from build123d import *

# Parameters (mm, degrees)
SKETCH1_W           = 153.67
SKETCH1_H           = 77.47
SKETCH1_R           = 2.667
SKETCH1_R_2         = 3.683
BOSS_EXTRUDE1_DEPTH = 6.096


with BuildPart() as part:
    # Sketch1 → Boss-Extrude1 (new body)
    with BuildSketch(Plane(origin=(0, 0, 0), x_dir=(1, 0, 0), z_dir=(0, 1, 0))):
        Rectangle(SKETCH1_W, SKETCH1_H)
        with Locations((-68.072, 29.972)):
            Circle(SKETCH1_R, mode=Mode.SUBTRACT)
        with Locations((-68.072, 14.732)):
            Circle(SKETCH1_R, mode=Mode.SUBTRACT)
        with Locations((-68.072, 0)):
            Circle(SKETCH1_R, mode=Mode.SUBTRACT)
        with Locations((-68.072, -29.972)):
            Circle(SKETCH1_R, mode=Mode.SUBTRACT)
        with Locations((-68.072, -16.256)):
            Circle(SKETCH1_R_2, mode=Mode.SUBTRACT)
        with Locations((-47.752, -29.972)):
            Circle(SKETCH1_R, mode=Mode.SUBTRACT)
        with Locations((-47.752, -16.256)):
            Circle(SKETCH1_R_2, mode=Mode.SUBTRACT)
        with Locations((-47.752, 0)):
            Circle(SKETCH1_R, mode=Mode.SUBTRACT)
        with Locations((-47.752, 14.732)):
            Circle(SKETCH1_R, mode=Mode.SUBTRACT)
        with Locations((-47.752, 29.972)):
            Circle(SKETCH1_R, mode=Mode.SUBTRACT)
        with Locations((-29.21, 29.972)):
            Circle(SKETCH1_R, mode=Mode.SUBTRACT)
        with Locations((-8.89, 29.972)):
            Circle(SKETCH1_R, mode=Mode.SUBTRACT)
        with Locations((-29.21, 8.89)):
            Circle(SKETCH1_R, mode=Mode.SUBTRACT)
        with Locations((-29.21, -8.89)):
            Circle(SKETCH1_R, mode=Mode.SUBTRACT)
        with Locations((-8.89, -29.972)):
            Circle(SKETCH1_R, mode=Mode.SUBTRACT)
        with Locations((-29.21, -29.972)):
            Circle(SKETCH1_R, mode=Mode.SUBTRACT)
        with Locations((-57.912, 20.066)):
            Circle(SKETCH1_R, mode=Mode.SUBTRACT)
        with Locations((-57.912, -20.066)):
            Circle(SKETCH1_R, mode=Mode.SUBTRACT)
        with Locations((-20.32, 20.066)):
            Circle(SKETCH1_R, mode=Mode.SUBTRACT)
        with Locations((-20.32, -20.066)):
            Circle(SKETCH1_R, mode=Mode.SUBTRACT)
        with Locations((-38.862, 20.066)):
            Circle(SKETCH1_R, mode=Mode.SUBTRACT)
        with Locations((-38.862, -20.066)):
            Circle(SKETCH1_R, mode=Mode.SUBTRACT)
        with Locations((20.32, -20.066)):
            Circle(SKETCH1_R, mode=Mode.SUBTRACT)
        with Locations((8.89, -29.972)):
            Circle(SKETCH1_R, mode=Mode.SUBTRACT)
        with Locations((29.21, -29.972)):
            Circle(SKETCH1_R, mode=Mode.SUBTRACT)
        with Locations((38.862, -20.066)):
            Circle(SKETCH1_R, mode=Mode.SUBTRACT)
        with Locations((47.752, -29.972)):
            Circle(SKETCH1_R, mode=Mode.SUBTRACT)
        with Locations((68.072, -29.972)):
            Circle(SKETCH1_R, mode=Mode.SUBTRACT)
        with Locations((68.072, 0)):
            Circle(SKETCH1_R, mode=Mode.SUBTRACT)
        with Locations((68.072, -16.256)):
            Circle(SKETCH1_R_2, mode=Mode.SUBTRACT)
        with Locations((57.912, -20.066)):
            Circle(SKETCH1_R, mode=Mode.SUBTRACT)
        with Locations((47.752, -16.256)):
            Circle(SKETCH1_R_2, mode=Mode.SUBTRACT)
        with Locations((29.21, -8.89)):
            Circle(SKETCH1_R, mode=Mode.SUBTRACT)
        with Locations((29.21, 8.89)):
            Circle(SKETCH1_R, mode=Mode.SUBTRACT)
        with Locations((57.912, 20.066)):
            Circle(SKETCH1_R, mode=Mode.SUBTRACT)
        with Locations((68.072, 14.732)):
            Circle(SKETCH1_R, mode=Mode.SUBTRACT)
        with Locations((68.072, 29.972)):
            Circle(SKETCH1_R, mode=Mode.SUBTRACT)
        with Locations((47.752, 14.732)):
            Circle(SKETCH1_R, mode=Mode.SUBTRACT)
        with Locations((47.752, 0)):
            Circle(SKETCH1_R, mode=Mode.SUBTRACT)
        with Locations((38.862, 20.066)):
            Circle(SKETCH1_R, mode=Mode.SUBTRACT)
        with Locations((20.32, 20.066)):
            Circle(SKETCH1_R, mode=Mode.SUBTRACT)
        with Locations((8.89, 29.972)):
            Circle(SKETCH1_R, mode=Mode.SUBTRACT)
        with Locations((29.21, 29.972)):
            Circle(SKETCH1_R, mode=Mode.SUBTRACT)
        with Locations((47.752, 29.972)):
            Circle(SKETCH1_R, mode=Mode.SUBTRACT)
        with BuildLine():
            Line((13.716, 14.986), (-13.716, 14.986))
            ThreePointArc((-13.716, 14.986), (-18.206128061, 13.126128061), (-20.066, 8.636))
            Line((-20.066, 8.636), (-20.066, -8.636))
            ThreePointArc((-20.066, -8.636), (-18.206128061, -13.126128061), (-13.716, -14.986))
            Line((-13.716, -14.986), (13.716, -14.986))
            ThreePointArc((13.716, -14.986), (18.206128061, -13.126128061), (20.066, -8.636))
            Line((20.066, -8.636), (20.066, 8.636))
            ThreePointArc((20.066, 8.636), (18.206128061, 13.126128061), (13.716, 14.986))
        make_face(mode=Mode.SUBTRACT)
    extrude(amount=BOSS_EXTRUDE1_DEPTH)


solid = part.part
Design review of the part built by this model. Coordinates are the model's own, in mm. A direction names the side the tool comes from. Coordinates: 2 decimals unless noted, no trailing zeros. Loops run counter-clockwise (first coordinate to the right, second up) from the corner with the lowest first, then second, coordinate; pieces in that order, holes last. Notation, with made-up numbers: (82, 38.25) -> (141, 38.25) arc R36 cw to (141, 74.25) -> close; hole circle Ø11 at (85.25, 37). An arc over 180 degrees is marked (long way). Use a Markdown table: item, result. Add a question column.
Item 1: Machinability: for faces 4 (the flat face through (20.066, 3, 0)), 5 (the flat face through (-1, 6.096, -18)), which of the approach directions +Z, -Z, +X, -X, +Y, -Y give a long, thin tool a straight path to every point of the face, cutting with its end or side? Answer none if there is none.
Item 2: We need section B-B, the plane z = 0. Write out the cut boundary in (x, y) (3 decimals), and give its area (3 significant figures).
Item 3: The part is to be moulded in two halves that separate along Z. For faces 1 (the flat face through (-76.835, 3, 1)), 2 (the cylindrical face through (49.19, 3.01, -32.22)), 3 (the cylindrical face through (36.746, 3.005, 21.689)), say which applies: +Z half, -Z half, draft (parallel to the pull), parting line (faces both ways), or undercut.
Item 4: We need section A-A, the plane x = -8.89. Write out the cut boundary in (y, z) (3 decimals), and give its area (3 significant figures).
Item 5: We need section D-D, the plane x = 39. Write out the cut boundary in (y, z) (3 decimals).
Item 6: Clearance check with a flat-ended pin moving along its axis: P1, Ø6, axis at x = -47.752, z = -14.732, coming from the +Y side. State where the tip first meets the part, or that it passes through.
Item 7: We need section C-C, the plane x = -29. Write out the cut boundary in (y, z) (3 decimals).
Item 8: Wall thickness on L1, parallel to X at y = 4, z = 16.5 (3 decimals); L2, parallel to X at y = 2, z = -8.89 (3 decimals); L3, parallel to Z at x = 1, y = 1.75 (3 decimals): over which ranges is each line inside the solid? List them lowest first. Write a range as from..to.
Numbers:
| question | item | result |
|---|---|---|
| 1 | face 4 | +Y, -Y |
| 1 | face 5 | +Z, -Z, +X, -X, +Y |
| 2 | outline | (-76.835, 0) -> (-70.739, 0) -> (-70.739, 6.096) -> (-76.835, 6.096) -> close; (-65.405, 0) -> (-50.419, 0) -> (-50.419, 6.096) -> (-65.405, 6.096) -> close; (-45.085, 0) -> (-20.066, 0) -> (-20.066, 6.096) -> (-45.085, 6.096) -> close; (20.066, 0) -> (45.085, 0) -> (45.085, 6.096) -> (20.066, 6.096) -> close; (50.419, 0) -> (65.405, 0) -> (65.405, 6.096) -> (50.419, 6.096) -> close; (70.739, 0) -> (76.835, 0) -> (76.835, 6.096) -> (70.739, 6.096) -> close |
| 2 | area | 562 mm^2 |
| 3 | face 1 | draft |
| 3 | face 2 | undercut |
| 3 | face 3 | undercut |
| 4 | outline | (0, -38.735) -> (6.096, -38.735) -> (6.096, -32.639) -> (0, -32.639) -> close; (0, -27.305) -> (6.096, -27.305) -> (6.096, -14.986) -> (0, -14.986) -> close; (0, 14.986) -> (6.096, 14.986) -> (6.096, 27.305) -> (0, 27.305) -> close; (0, 32.639) -> (6.096, 32.639) -> (6.096, 38.735) -> (0, 38.735) -> close |
| 4 | area | 225 mm^2 |
| 5 | outline | (0, -38.735) -> (6.096, -38.735) -> (6.096, -22.729) -> (0, -22.729) -> close; (0, -17.403) -> (6.096, -17.403) -> (6.096, 17.403) -> (0, 17.403) -> close; (0, 22.729) -> (6.096, 22.729) -> (6.096, 38.735) -> (0, 38.735) -> close |
| 6 | P1 | stops at y = 6.1 |
| 7 | outline | (0, -38.735) -> (6.096, -38.735) -> (6.096, -32.631) -> (0, -32.631) -> close; (0, -27.313) -> (6.096, -27.313) -> (6.096, -11.549) -> (0, -11.549) -> close; (0, -6.231) -> (6.096, -6.231) -> (6.096, 6.231) -> (0, 6.231) -> close; (0, 11.549) -> (6.096, 11.549) -> (6.096, 27.313) -> (0, 27.313) -> close; (0, 32.631) -> (6.096, 32.631) -> (6.096, 38.735) -> (0, 38.735) -> close |
| 8 | L1 | x = -76.835..-71.747, -64.397..-51.427, -44.077..44.077, 51.427..64.397, 71.747..76.835 |
| 8 | L2 | x = -76.835..-31.877, -26.543..-20.061, 20.061..26.543, 31.877..76.835 |
| 8 | L3 | z = -38.735..-14.986, 14.986..38.735 |
